```python
from build123d import *

# Parameters (mm, degrees)
BOSS_EXTRUDE1_DEPTH   = 38
BOSS_EXTRUDE1_2_DEPTH = 38
SKETCH2_W             = 42.2
SKETCH2_H             = 5.9
BOSS_EXTRUDE2_DEPTH   = 2
BOSS_EXTRUDE3_DEPTH   = 18
SKETCH4_W             = 42.2
SKETCH4_H             = 40
BOSS_EXTRUDE4_DEPTH   = 2
SKETCH5_W             = 38.2
SKETCH5_H             = 11.95
CUT_EXTRUDE1_DEPTH    = 81.281509747
SKETCH6_W             = 2
SKETCH6_H             = 10
BOSS_EXTRUDE5_DEPTH   = 2
SKETCH7_W             = 2
SKETCH7_H             = 10
BOSS_EXTRUDE6_DEPTH   = 2
SKETCH8_W             = 10
SKETCH8_H             = 2
BOSS_EXTRUDE7_DEPTH   = 2


with BuildPart() as part:
    # Sketch1 → Boss-Extrude1 (new body)
    with BuildSketch(Plane(origin=(0, 0, 0), x_dir=(1, 0, 0), z_dir=(0, 1, 0))):
        Polygon((-62.898983402, -26.09346473), (-62.898983402, -24.19346473), (-60.898983402, -24.19346473), (-60.898983402, -22.19346473), (-64.898983402, -22.19346473), (-64.898983402, -28.09346473), (-60.898983402, -28.09346473), (-60.898983402, -26.09346473), align=None)
    extrude(amount=BOSS_EXTRUDE1_DEPTH)



with BuildPart() as body_2:
    # Sketch1 → Boss-Extrude1 2 (new body)
    with BuildSketch(Plane(origin=(0, 0, 0), x_dir=(1, 0, 0), z_dir=(0, 1, 0))):
        Polygon((-26.698983402, -22.19346473), (-26.698983402, -24.19346473), (-24.698983402, -24.19346473), (-24.698983402, -26.09346473), (-26.698983402, -26.09346473), (-26.698983402, -28.09346473), (-22.698983402, -28.09346473), (-22.698983402, -22.19346473), align=None)
    extrude(amount=BOSS_EXTRUDE1_2_DEPTH)


with BuildPart() as part_1:
    add(part.part)

    add(body_2.part)  # Boss-Extrude2 merges body 2
    # Sketch2 → Boss-Extrude2 (add)
    with BuildSketch(Plane(origin=(0, 0, 0), x_dir=(1, 0, 0), z_dir=(0, 1, 0))):
        with Locations((-43.798983402, -25.14346473)):
            Rectangle(SKETCH2_W, SKETCH2_H)
    extrude(amount=-BOSS_EXTRUDE2_DEPTH)

    # Sketch3 → Boss-Extrude3 (add)
    with BuildSketch(Plane(origin=(0, 0, 22.19346473), x_dir=(-1, 0, 0), z_dir=(0, 0, -1))):
        Polygon((24.698983402, 38), (22.698983402, 38), (22.698983402, -2), (64.898983402, -2), (64.898983402, 38), (62.898983402, 38), (62.898983402, 0), (24.698983402, 0), align=None)
    extrude(amount=BOSS_EXTRUDE3_DEPTH)

    # Sketch4 → Boss-Extrude4 (add)
    with BuildSketch(Plane(origin=(0, 0, 4.19346473), x_dir=(-1, 0, 0), z_dir=(0, 0, -1))):
        with Locations((43.798983402, 18)):
            Rectangle(SKETCH4_W, SKETCH4_H)
    extrude(amount=BOSS_EXTRUDE4_DEPTH)

    # Sketch5 → Cut-Extrude1 (cut, through all)
    with BuildSketch(Plane(origin=(0, 0, 0), x_dir=(1, 0, 0), z_dir=(0, 1, 0))):
        with Locations((-43.798983402, -10.16846473)):
            Rectangle(SKETCH5_W, SKETCH5_H)
    extrude(amount=-CUT_EXTRUDE1_DEPTH, mode=Mode.SUBTRACT)

    # Sketch6 → Boss-Extrude5 (add)
    with BuildSketch(Plane(origin=(-60.898983402, 0, 0), x_dir=(0, 0, -1), z_dir=(1, 0, 0))):
        with Locations((-27.09346473, 24)):
            Rectangle(SKETCH6_W, SKETCH6_H)
        with Locations((-23.19346473, 24)):
            Rectangle(SKETCH6_W, SKETCH6_H)
        with Locations((-27.09346473, 14)):
            Rectangle(SKETCH6_W, SKETCH6_H)
        with Locations((-23.19346473, 14)):
            Rectangle(SKETCH6_W, SKETCH6_H)
    extrude(amount=BOSS_EXTRUDE5_DEPTH)

    # Sketch7 → Boss-Extrude6 (add)
    with BuildSketch(Plane.ZY.offset(26.698983402)):
        with Locations((27.09346473, 24)):
            Rectangle(SKETCH7_W, SKETCH7_H)
        with Locations((27.09346473, 14)):
            Rectangle(SKETCH7_W, SKETCH7_H)
        with Locations((23.19346473, 14)):
            Rectangle(SKETCH7_W, SKETCH7_H)
        with Locations((23.19346473, 24)):
            Rectangle(SKETCH7_W, SKETCH7_H)
    extrude(amount=BOSS_EXTRUDE6_DEPTH)

    # Sketch8 → Boss-Extrude7 (add)
    with BuildSketch(Plane(origin=(0, 0, 0), x_dir=(1, 0, 0), z_dir=(0, 1, 0))):
        with Locations((-48.798983402, -23.19346473)):
            Rectangle(SKETCH8_W, SKETCH8_H)
        with Locations((-38.798983402, -23.19346473)):
            Rectangle(SKETCH8_W, SKETCH8_H)
        with Locations((-48.798983402, -27.09346473)):
            Rectangle(SKETCH8_W, SKETCH8_H)
        with Locations((-38.798983402, -27.09346473)):
            Rectangle(SKETCH8_W, SKETCH8_H)
    extrude(amount=BOSS_EXTRUDE7_DEPTH)


solid = part_1.part
```
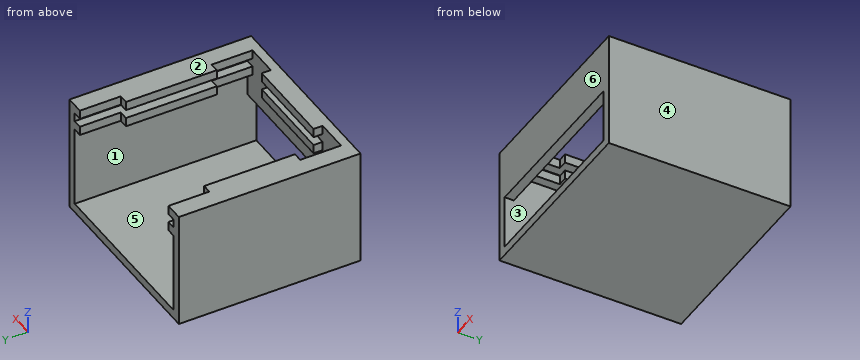
Model file for the job. Use its own axes, mm. Face numbers are marked on the shaded views. A direction names the side the tool comes from. Round coordinates to 2 decimals unless told otherwise and drop trailing zeros. Write each loop counter-clockwise with the first axis right and the second up, starting at its lowest first coordinate (ties: lowest second). Pieces come first, ordered by that corner, then holes. Notation, with made-up numbers: (19.25, -38) -> (36.25, -38) arc R11 ccw to (36.25, -18) -> close; hole circle Ø9 at (2.25, 1). An arc over 180 degrees is marked (long way). Answer as CSV lines item,"result".
1. Slice it at A-A, the plane x = -41.5. List the corners of the cut face in (y, z).
Resolved:
outline,"(-2, 2.19) -> (38, 2.19) -> (38, 4.19) -> (-2, 4.19) -> close; (-2, 16.14) -> (0, 16.14) -> (0, 22.19) -> (2, 22.19) -> (2, 24.19) -> (0, 24.19) -> (0, 26.09) -> (2, 26.09) -> (2, 28.09) -> (-2, 28.09) -> close"
2. Pin check, flat tips, straight feed: pin 1 Ø10 at (x, y) = (-57.5, 5.5) entering from +Z; pin 2 Ø1 at (x, z) = (-39.5, 27.5) entering from +Y; pin 3 Ø0.6 at (x, z) = (-27.5, 26.5) entering from +Y; pin 4 Ø1.5 at (x, y) = (-49, 20.5) entering from +Z. Stop position of each tip, or through.
Resolved:
pin 1,"z = 28.09"
pin 2,"y = 2"
pin 3,"y = 29"
pin 4,"z = 4.19"
3. Slice it at D-D, the plane z = 20.25. List the corners of the cut face in (x, y), plus the area to 3 significant figures.
Resolved:
outline,"(-64.9, -2) -> (-22.7, -2) -> (-22.7, 38) -> (-24.7, 38) -> (-24.7, 0) -> (-62.9, 0) -> (-62.9, 38) -> (-64.9, 38) -> close"
area,"236 mm²"
4. Mould opens along Z. For the marked faces 1, 2, 3 and 4 say: +Z half, -Z half, draft (parallel to the pull), parting line (faces both ways), or undercut.
Resolved:
face 1,"undercut"
face 2,"+Z half"
face 3,"undercut"
face 4,"draft"
5. Slice it at C-C, the plane y = 7.5. List the corners of the cut face in (x, z).
Resolved:
outline,"(-64.9, 2.19) -> (-22.7, 2.19) -> (-22.7, 28.09) -> (-26.7, 28.09) -> (-26.7, 26.09) -> (-24.7, 26.09) -> (-24.7, 24.19) -> (-26.7, 24.19) -> (-26.7, 22.19) -> (-24.7, 22.19) -> (-24.7, 4.19) -> (-62.9, 4.19) -> (-62.9, 22.19) -> (-60.9, 22.19) -> (-60.9, 24.19) -> (-62.9, 24.19) -> (-62.9, 26.09) -> (-60.9, 26.09) -> (-60.9, 28.09) -> (-64.9, 28.09) -> close"
6. Slice it at B-B, the plane z = 10. List the corners of the cut face in (x, y), plus the area to 3 significant figures.
Resolved:
outline,"(-64.9, -2) -> (-62.9, -2) -> (-62.9, 38) -> (-64.9, 38) -> close; (-24.7, -2) -> (-22.7, -2) -> (-22.7, 38) -> (-24.7, 38) -> close"
area,"160 mm²"
7. Drill centre lines: line 1 (Z direction, x = -61.5, y = 11); line 2 (X direction, y = 29.5, z = 12.5); line 3 (Z direction, x = -39, y = 13.5). Where is each one in solid material? Low to high.
Resolved:
line 1,"2.19 to 4.19, 22.19 to 24.19, 26.09 to 28.09"
line 2,"-64.9 to -62.9, -24.7 to -22.7"
line 3,"2.19 to 4.19"
8. Tool access for the marked faces 5 and 6: list every direction of +Z, -Z, +X, -X, +Y, -Y with a clear straight run to the whole face (end or side of a thin tool).
Resolved:
face 5,"+Y, -Y"
face 6,"+Z, -Z, +X, -X, -Y"
